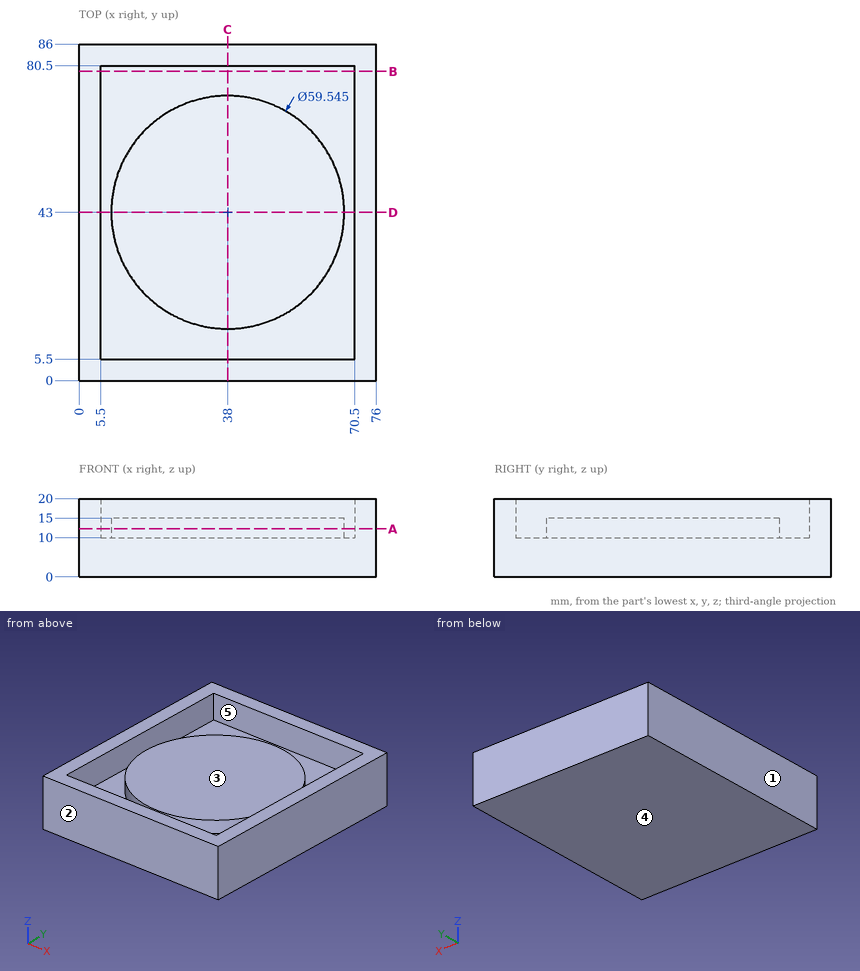
Check sheet for the drawn part. Datum: minimum x, y, z corner. Units: mm. A direction names the side the tool comes from. Round coordinates to 2 decimals unless told otherwise and drop trailing zeros. Write each loop counter-clockwise with the first axis right and the second up, starting at its lowest first coordinate (ties: lowest second). Pieces come first, ordered by that corner, then holes. Notation, with made-up numbers: (84.25, 87.5) - (103.25, 87.5) arc R21 ccw to (103.25, 102.5) - close; hole circle Ø9 at (39, -31). An arc over 180 degrees is marked (long way). Return JSON: item names as keys, results as strings.
Q1. Depth check by flat-ended pin: P1, Ø1.5, axis at x = 68, y = 25.5, coming from the +Z side; P2, Ø10, axis at x = 34.5, z = 9, coming from the -Y side; P3, Ø6, axis at x = 9.5, y = 53, coming from the +Z side. Enter the tip coordinate at first touch or a pass-through.
Returned:
{"P1": "stops at z = 10", "P2": "stops at y = 0", "P3": "stops at z = 15"}
Q2. Draft check along Y on the marked faces 1, 2 and 3. Enter one of: released by +Y, released by -Y, zero draft, split by the parting line, or undercut.
Returned:
{"face 1": "zero draft", "face 2": "released by -Y", "face 3": "undercut"}
Q3. Cross-section at B-B (y = 79). Record the boundary of the cut face in (x, z).
Returned:
{"outline": "(0, 0) - (76, 0) - (76, 20) - (70.5, 20) - (70.5, 10) - (5.5, 10) - (5.5, 20) - (0, 20) - close"}
Q4. Cross-section at A-A (z = 12.25). Record the boundary of the cut face in (x, y) (1 decimal), then the cut area to 3 significant figures.
Returned:
{"outline": "(0, 0) - (76, 0) - (76, 86) - (0, 86) - close; circle Ø59.5 at (38, 43); hole (5.5, 5.5) - (70.5, 5.5) - (70.5, 80.5) - (5.5, 80.5) - close", "area": "4,450 mm²"}
Q5. Cross-section at C-C (x = 38). Record the boundary of the cut face in (y, z), then the cut area to 3 significant figures.
Returned:
{"outline": "(0, 0) - (86, 0) - (86, 20) - (80.5, 20) - (80.5, 10) - (72.77, 10) - (72.77, 15) - (13.23, 15) - (13.23, 10) - (5.5, 10) - (5.5, 20) - (0, 20) - close", "area": "1,270 mm²"}
Q6. Scan lines: L1, parallel to Y at x = 60.5, z = 16.75; L2, parallel to Y at x = 38.5, z = 11; L3, parallel to X at y = 55, z = 12.5. Record each from-to range of solid material in increasing order. Write a range as from..to.
Returned:
{"L1": "y = 0..5.5, 80.5..86", "L2": "y = 0..5.5, 13.23..72.77, 80.5..86", "L3": "x = 0..5.5, 10.75..65.25, 70.5..76"}
Q7. Cross-section at D-D (y = 43). Record the boundary of the cut face in (x, z).
Returned:
{"outline": "(0, 0) - (76, 0) - (76, 20) - (70.5, 20) - (70.5, 10) - (67.77, 10) - (67.77, 15) - (8.23, 15) - (8.23, 10) - (5.5, 10) - (5.5, 20) - (0, 20) - close"}
Q8. Access from +Z, -Z, +X, -X, +Y, -Y to the whole of each face (thin tool, end or side, straight path). Record for the marked faces 4 and 5.
Returned:
{"face 4": "-Z, +X, -X, +Y, -Y", "face 5": "+Z"}
